Autodesk Fusion 360 part; units mm, degrees
sketch "Sketch1" plane through (0, 0, 0) normal (0, 1, 0) x (1, 0, 0)
  line L0 (-90.5, 11) -> (80.5, 11)
  line L1 (80.5, 11) -> (80.5, -11)
  line L2 (80.5, -11) -> (-90.5, -11)
  line L3 (-90.5, -11) -> (-90.5, 11)
  circle A0 centre (-71.5, 0) radius 1.65
  circle A1 centre (-79.5, 8) radius 1.65
  circle A2 centre (-87.5, 0) radius 1.65
  circle A3 centre (-79.5, -8) radius 1.65
  circle A4 centre (70.5, 0) radius 2.75
  point P0 (-79.5, 0)
  dimension "d6" = 11
  dimension "d7" = 22
  dimension "d10" = 3.3
  dimension "d11" = 8
  dimension "d13" = 360
  dimension "d14" = 5.5
  dimension "d15" = 10
  dimension "d16" = 150
  dimension "d17" = 11
  dimension "d18" = 11
  dimension "d19" = 11
extrude "Extrude1" add sketch "Sketch1" along normal blind 4
fillet "Fillet1" radius 11 2 edges at (80.5, 2, -11) (80.5, 2, 11)
fillet "Fillet2" radius 11 2 edges at (-90.5, 2, 11) (-90.5, 2, -11)
sketch "Sketch3" plane through (0, 4, 0) normal (0, 1, 0) x (-1, 0, 0)
  circle A0 centre (79.5, -8) radius 1.65
  circle A1 centre (87.5, 0) radius 1.65
  circle A2 centre (79.5, 8) radius 1.65
  circle A3 centre (-70.5, 0) radius 2.75
  circle A4 centre (71.5, 0) radius 1.65
  arc A5 (79.5, -11) -> (79.5, 11) centre (79.5, 0) ccw
  line L0 (79.5, 11) -> (-69.5, 11)
  arc A6 (-69.5, 11) -> (-69.5, -11) centre (-69.5, 0) ccw
  line L1 (-69.5, -11) -> (79.5, -11)
  line L2 (27, 4) -> (-13, 4)
  arc A7 (-13, 4) -> (-13, -4) centre (-13, 0) ccw
  line L3 (-13, -4) -> (27, -4)
  arc A8 (27, -4) -> (27, 4) centre (27, 0) ccw
  line L4 (27, 0) -> (-13, 0) construction
  dimension "d24" = 8
  dimension "d30" = 40
extrude "Extrude2" cut sketch "Sketch3" against normal up to surface (4 mm away) contours L2 A7 L3 A8
sketch "Sketch4" plane through (0, 4, 0) normal (0, 1, 0) x (-1, 0, 0)
  line L0 (27, -4) -> (-13, -4)
  arc A0 (-13, 4) -> (-13, -4) centre (-13, 0) ccw
  line L1 (-13, 4) -> (27, 4)
  arc A1 (27, -4) -> (27, 4) centre (27, 0) ccw
  circle A2 centre (79.5, -8) radius 1.65
  circle A3 centre (87.5, 0) radius 1.65
  circle A4 centre (79.5, 8) radius 1.65
  circle A5 centre (-70.5, 0) radius 2.75
  circle A6 centre (71.5, 0) radius 1.65
  arc A7 (79.5, -11) -> (79.5, 11) centre (79.5, 0) ccw
  line L2 (79.5, 11) -> (-69.5, 11)
  arc A8 (-69.5, 11) -> (-69.5, -11) centre (-69.5, 0) ccw
  line L3 (-69.5, -11) -> (79.5, -11)
  circle A9 centre (79.5, 0) radius 1.5
  dimension "d27" = 3
extrude "Extrude3" cut sketch "Sketch4" against normal up to surface (4 mm away) contours A9
equation "length = 150 mm"
equation "width = 22 mm"
equation "thickness = 4 mm"
equation "d5 = length + width / 2"
equation "d6 = width / 2"
equation "d7 = width"
equation "d16 = length"
equation "d17 = width / 2"
equation "d18 = width / 2"
equation "d20 = thickness"
equation "d22 = width / 2"
equation "d23 = width / 2"
For this review, take the finished solid that the model builds, in its own axes (mm). A direction names the side the tool comes from. Give positions to 0.01 mm unless a question says otherwise; leave off trailing zeros. Loops run counter-clockwise (first coordinate to the right, second up) from the corner with the lowest first, then second, coordinate; pieces in that order, holes last.
Item 1: Take a section at C-C, the plane z = 8. State the section outline as (x, y) points.
Item 2: Take a section at B-B, the plane y = 1.15. Give the number of separate pieces and of enclosed holes in the cut face, and give its area (3 significant figures).
Item 3: Tool access review of faces 1 (the flat face through (-7, 2, -4)), 2 (the flat face through (-4, 2, 11)): name each direction out of +Z, -Z, +X, -X, +Y, -Y from which nothing blocks a thin tool from reaching the whole face with its end or side.
Item 4: For line 1 along Z through (x, y) = (-79.5, 2.15); line 2 along Z through (x, y) = (-15, 2.95); line 3 along X through (y, z) = (1.3, -1.75), list the stretches that pass through material, from the lowest coordinate up.
Item 5: Insertion check: pin 1 (3 mm diameter, centred on x = -79.5, z = 8, fed in from -Y); pin 2 (1 mm diameter, centred on y = 1, z = -4, fed in from +X). Each pin has a flat end and moves straight along its axis. Give the tip position at first contact, or say it passes through.
Item 6: Take a section at A-A, the plane x = -21.5. State the section outline as (y, z) points, and give its area (3 significant figures).
Item 7: Draft analysis for pull direction Z (two halves, no side actions). For faces 3 (the cylindrical face through (77.193, 2.028, 7.864)), 4 (the cylindrical face through (17, 2, 0)), 5 (the flat face through (-6, 0, -5)), state which applies: +Z half, -Z half, draft (parallel to the pull), parting line (faces both ways), or undercut.
Calculated:
1. outline: (-87.05, 0) - (-81.15, 0) - (-81.15, 4) - (-87.05, 4) - close; (-77.85, 0) - (77.05, 0) - (77.05, 4) - (-77.85, 4) - close
2. separate pieces: 1
2. enclosed holes: 7
2. area: 3,220 mm2
3. face 1: +Y, -Y
3. face 2: +Z, +X, -X, +Y, -Y
4. line 1: z = -11 to -9.65, -6.35 to -1.5, 1.5 to 6.35, 9.65 to 11
4. line 2: z = -11 to -4, 4 to 11
4. line 3: x = -90.36 to -30.6, 16.6 to 68.38, 72.62 to 80.36
5. pin 1: passes through
5. pin 2: stops at x = 79.93
6. outline: (0, -11) - (4, -11) - (4, -4) - (0, -4) - close; (0, 4) - (4, 4) - (4, 11) - (0, 11) - close
6. area: 56.0 mm2
7. face 3: +Z half
7. face 4: undercut
7. face 5: draft
